Can you work these out from the model? Positions are in its coordinate system, mm. Face numbers are marked on the shaded views. A direction names the side the tool comes from. Coordinates: 2 decimals unless noted, no trailing zeros. Order: outer loops, then holes, each group sorted by start corner. A loop starts at its lowest first (then second) coordinate and runs counter-clockwise, first axis right, second up. Notation, with made-up numbers: (24, -1) -> (29, -1) arc R36 ccw to (29, 37) -> close; hole circle Ø4 at (39.5, 82). An arc over 180 degrees is marked (long way). Answer as a JSON object with one key per item and string values. Group by question number.
(1) I want a section at B-B, the plane z = 16.5. State how many separate pieces and enclosed holes the cut face has, plus the area to 3 significant figures.
(2) I want a section at D-D, the plane x = -65. List the corners of the cut face in (y, z) for me, plus the area to 3 significant figures.
(3) I want a section at A-A, the plane y = 0. List the corners of the cut face in (x, z) for me.
(4) For pin 1 (6 mm diameter, centred on y = -24, z = 4, fed in from -X); pin 2 (1 mm diameter, centred on y = 43, z = 8, fed in from -X); pin 3 (7 mm diameter, centred on x = 4, z = 4.5, fed in from +Y); pin 4 (5.5 mm diameter, centred on x = -55, y = -40, fed in from -Z), each with a flat end and sliding along its axis, tell me the tip position at first contact or that it passes through.
(5) I want a section at C-C, the plane x = 96.5. List the corners of the cut face in (y, z) for me, plus the area to 3 significant figures.
(6) I need wall thicknesses on line 1 (Y direction, x = 0.08, z = 15.75); line 2 (Y direction, x = -55, z = 10); line 3 (X direction, y = -9.5, z = 15.25). Which ranges of each line are inside material? Lowest first, please.
(7) If we mould it in two halves opening along Y, with no side actions, what happens to the marked faces 4, 5 and 6? For each: pulls with the +Y half, pulls with the -Y half, needs draft (parallel to the pull), parting line crosses it, or undercut.
(8) Which directions (+Z, -Z, +X, -X, +Y, -Y) give clear straight access to the entire face, cutting with the end or side of a thin tool? Please do the marked faces 1, 2 and 3.
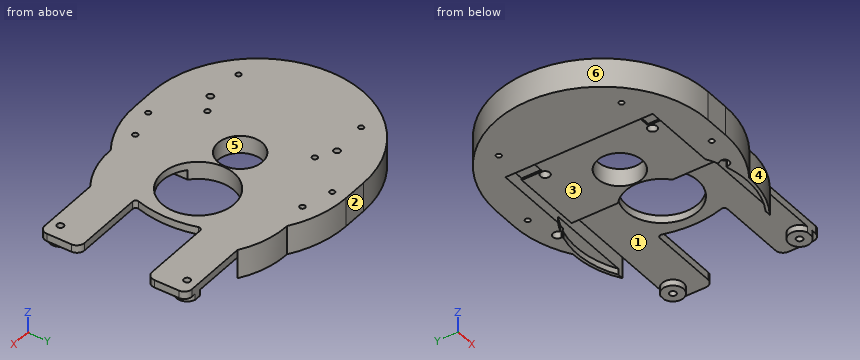
Autodesk Inventor part; units mm, degrees
ref_plane "YZ Plane" through (0, 0, 0) normal (1, 0, 0) x (0, 1, 0)
ref_plane "XZ Plane" through (0, 0, 0) normal (0, 1, 0) x (-1, 0, 0)
ref_plane "XY Plane" through (0, 0, 0) normal (0, 0, 1) x (1, 0, 0)
sketch "Sketch1" plane through (0, 0, 0) normal (0, 0, 1) x (1, 0, 0)
  line L0 (-19.2849, 35) -> (-19.2849, -35) construction
  line L1 (19.7114, 54.5) -> (19.7114, -54.5) construction
  line L2 (-19.2849, 35) -> (19.7114, 54.5) construction
  line L3 (-19.2849, -35) -> (19.7114, -54.5) construction
  circle A0 centre (0.08, 0) radius 14.5
  line L4 (-19.2849, 35) -> (0.08, 0) construction
  line L5 (0.08, 0) -> (-19.2849, -35) construction
  circle A1 centre (19.7114, 54.5) radius 1.75
  circle A2 centre (-19.2849, 35) radius 1.75
  circle A3 centre (-19.2849, -35) radius 1.75
  circle A4 centre (19.7114, -54.5) radius 1.75
  line L6 (-16, -69) -> (0, -69)
  line L7 (0, 69) -> (-16, 69)
  arc A5 (-16, 69) -> (-16, -69) centre (-16, 0) ccw
  arc A6 (0, -69) -> (0, 69) centre (0, 0) ccw
  line L8 (-85, 0) -> (69, 0) construction
  circle A7 centre (-19.2849, 35) radius 3
  circle A8 centre (-19.2849, -35) radius 3
  circle A9 centre (19.7114, 54.5) radius 3
  circle A10 centre (19.7114, -54.5) radius 3
  line L9 (0, -60) -> (0, 60) construction
  line L10 (-55, 40) -> (-55, -40) construction
  circle A11 centre (-55, 40) radius 1.65
  circle A12 centre (-55, -40) radius 1.65
  circle A13 centre (0, -60) radius 1.65
  circle A14 centre (0, 60) radius 1.65
  point P0 (-19.2849, 0)
  point P1 (19.7114, 0)
  point P2 (-55, 0)
  dimension "d0" = 70
  dimension "d1" = 109
  dimension "d2" = 43.6
  dimension "d3" = 29
  dimension "d4" = 40
  dimension "d5" = 3.5
  dimension "d7" = 138
  dimension "d8" = 154
  dimension "d33" = 6
  dimension "d55" = 85.08
  dimension "d110" = 120
  dimension "d111" = 30
  dimension "d112" = 80
  dimension "d113" = 3.3
extrude "Extrusion1" add sketch "Sketch1" along normal blind 19 contours A5 L7 A6 L6 | A7 | A8 | A9 | A10 | A11 | A12 | A13 | A14
sketch "Sketch2" plane through (0, 0, 19) normal (0, 0, 1) x (1, 0, 0)
  circle A0 centre (-52.47, 0) radius 18.5329 construction
  circle A1 centre (-71.0029, 0) radius 2
  circle A2 centre (-43.2035, 16.05) radius 2
  circle A3 centre (-43.2035, -16.05) radius 2
  circle A4 centre (0.08, 0) radius 14.5
  circle A5 centre (19.7114, -54.5) radius 1.75
  circle A6 centre (-19.2849, -35) radius 1.75
  circle A7 centre (-19.2849, 35) radius 1.75
  circle A8 centre (19.7114, 54.5) radius 1.75
  line L0 (-16, -69) -> (0, -69)
  arc A9 (0, -69) -> (0, 69) centre (0, 0) ccw
  line L1 (0, 69) -> (-16, 69)
  arc A10 (-16, 69) -> (-16, -69) centre (-16, 0) ccw
  arc A11 (-16, 69) -> (-16, -69) centre (-16, 0) ccw construction
  line L2 (-85, 0) -> (69, 0) construction
  circle A12 centre (-43.2035, -16.05) radius 5
  circle A13 centre (-43.2035, 16.05) radius 5
  circle A14 centre (-71.0029, 0) radius 5
  dimension "d11" = 120
  dimension "d12" = 120
  dimension "d13" = 32.1
  dimension "d14" = 52.55
  dimension "d40" = 4
  dimension "d49" = 10
sketch "Sketch3" plane through (0, 0, 0) normal (0, 0, -1) x (-1, 0, 0)
  circle A0 centre (30.8533, 41.3) radius 2.1
  circle A1 centre (-0.08, 0) radius 14.5
  circle A2 centre (30.8533, -41.3) radius 2.1
  line L0 (30.8533, 41.3) -> (-0.08, 0) construction
  line L1 (-0.08, 0) -> (30.8533, -41.3) construction
  circle A3 centre (-0.08, 0) radius 14.5 construction
  circle A4 centre (-19.7114, -54.5) radius 1.75 construction
  circle A5 centre (19.2849, -35) radius 1.75 construction
  circle A6 centre (19.2849, 35) radius 1.75 construction
  circle A7 centre (-19.7114, 54.5) radius 1.75 construction
  line L2 (16, -69) -> (0, -69) construction
  arc A8 (16, -69) -> (16, 69) centre (16, 0) ccw construction
  line L3 (0, 69) -> (16, 69) construction
  arc A9 (0, 69) -> (0, -69) centre (0, 0) ccw construction
  arc A10 (16, -69) -> (16, 69) centre (16, 0) ccw construction
  line L4 (85, 0) -> (-69, 0) construction
  arc A11 (0, 69) -> (0, -69) centre (0, 0) ccw construction
  line L5 (30.8533, 41.3) -> (30.8533, -41.3)
  line L6 (37.5533, 48) -> (-142.6467, 48)
  line L7 (-142.6467, 48) -> (-142.6467, -48)
  line L8 (-142.6467, -48) -> (37.5533, -48)
  line L9 (37.5533, -48) -> (37.5533, 48)
  line L10 (30.8533, 41.3) -> (37.5533, 41.3) construction
  line L11 (30.8533, 41.3) -> (30.8533, 48) construction
  line L12 (30.8533, -41.3) -> (37.5533, -41.3) construction
  line L13 (30.8533, -41.3) -> (30.8533, -48) construction
  circle A12 centre (-107.4467, 41.3) radius 2.1
  circle A13 centre (-107.4467, -41.3) radius 2.1
  line L14 (30.8533, 41.3) -> (-107.4467, 41.3) construction
  line L15 (30.8533, -41.3) -> (-107.4467, -41.3) construction
  line L16 (-23.4467, 48) -> (-23.4467, -48)
  circle A14 centre (-38.88, 0) radius 23.5
  circle A15 centre (-38.88, 0) radius 55.5
  arc A16 (-38.1482, 57.4953) -> (-70.5383, 48) centre (-38.88, 0) ccw
  arc A17 (-70.5383, -48) -> (-38.1482, -57.4953) centre (-38.88, 0) ccw
  line L17 (-38.1482, 57.4953) -> (-38.1482, 48)
  line L18 (-70.5383, 48) -> (-38.1482, 48)
  line L19 (-38.1482, -57.4953) -> (-38.1482, -48)
  line L20 (-70.5383, -48) -> (-38.1482, -48)
  dimension "d15" = 51.6
  dimension "d18" = 82.6
  dimension "d20" = 180.2
  dimension "d22" = 96
  dimension "d29" = 138.3
  dimension "d59" = 4.2
  dimension "d61" = 61
  dimension "d68" = 47
  dimension "d69" = 38.8
  dimension "d70" = 69
  dimension "d118" = 111
  dimension "d141" = 2
extrude "Extrusion14" cut sketch "Sketch3" against normal blind 14 contours L16 A14 L8 A15 L6 | L16 A14 | A15 L8 L7 L6 picked at (-49.8352, 39.5964) picked at (-36.3678, -0.9407)
extrude "Extrusion15" cut sketch "Sketch3" against normal blind 7.5 contours L6 A15 L8 L16 A14 | L6 L9 L8 A15 | A14 L16 picked at (-10.5973, 24.5754) picked at (-22.3115, -4.6826)
extrude "Extrusion16" cut sketch "Sketch3" against normal through all contours A0 | A2
sketch "Sketch8" plane through (0, 0, 19) normal (0, 0, 1) x (1, 0, 0)
  line L0 (-37.5533, 48) -> (-37.5533, -48)
  circle A0 centre (107.4467, -41.3) radius 2.1
  circle A1 centre (107.4467, 41.3) radius 2.1
  line L1 (-37.5533, -48) -> (117.4467, -48)
  line L2 (117.4467, -48) -> (117.4467, -22)
  line L3 (117.4467, -22) -> (-37.5533, -22)
  line L4 (-37.5533, -22) -> (-37.5533, -48)
  line L5 (49.5681, 48) -> (-37.5533, 48)
  line L6 (-37.5533, 48) -> (117.4467, 48)
  line L7 (117.4467, 48) -> (117.4467, 22)
  line L8 (117.4467, 22) -> (-37.5533, 22)
  line L9 (-37.5533, 22) -> (-37.5533, 48)
  circle A2 centre (107.4467, -41.3) radius 2.1
  circle A3 centre (107.4467, 41.3) radius 2.1
  arc A4 (109.474, -48) -> (105.4194, -48) centre (107.4467, -41.3) ccw
  arc A5 (105.4194, 48) -> (109.474, 48) centre (107.4467, 41.3) ccw
  point P0 (122.0315, -50.7282)
  point P1 (122.0315, 31.8718)
  dimension "d79" = 26
  dimension "d80" = 155
  dimension "d81" = 14
extrude "Extrusion18" add sketch "Sketch8" against normal up to surface (5 mm away)
extrude "Extrusion19" add sketch "Sketch8" against normal blind 9 contours L6 A5 | A4 L1
extrude "Extrusion17" cut sketch "Sketch3" against normal through all contours A14 L16 | L16 A14
extrude "Extrusion20" cut sketch "Sketch3" against normal through all contours A0 | A2
extrude "Extrusion21" cut sketch "Sketch1" along normal through all contours A2 | A3
extrude "Extrusion22" cut sketch "Sketch1" along normal blind 14 contours A7 | A8 | A9 | A10
extrude "Extrusion23" cut sketch "Sketch1" along normal through all contours A11 | A12 | A13 | A14
fillet "Fillet1" radius 5 1 edges at (117.4467, 48, 16.5)
fillet "Fillet2" radius 5 3 edges at (117.4467, 22, 16.5) (117.4467, -22, 16.5) (117.4467, -48, 16.5)
thread "Thread1"
thread "Thread2"
thread "Thread3"
thread "Thread4"
thread "Thread6"
thread "Thread7"
thread "Thread8"
thread "Thread9"
fillet "Fillet3" radius 2 2 edges at (65.3988, 22, 16.5) (65.3988, -22, 16.5)
extrude "Extrusion27" add sketch "Sketch3" against normal up to surface (19 mm away) contours L6 A15 L17 | L6 A16 L17 A15 | A15 L19 A17 L8 | L8 L19 A15 picked at (-54.2009, 49.4023) picked at (-54.2009, -49.4023)
extrude "Extrusion26" cut sketch "Sketch3" against normal blind 4 contours L16 A14 L8 A15 L6 | L6 L17 A15 | L6 A15 L8 L16 A14 | L6 A15 L17 | L8 L19 A15 | A15 L19 L8
chamfer "Chamfer2" distance 1 angle 45 4 edges at (22.2868, 52.9615, 2) (18.6661, 51.688, 2) (18.6661, -51.688, 2) (22.2868, -52.9615, 2)
sketch "Sketch10" plane through (0, 0, 7.5) normal (0, 0, -1) x (-1, 0, 0)
  line L0 (37.5533, 48) -> (37.5533, -48)
  line L1 (37.5533, 48) -> (22.5533, 48)
  line L2 (22.5533, 48) -> (22.5533, 34.5)
  line L3 (22.5533, 34.5) -> (37.5533, 34.5)
  line L4 (37.5533, 34.5) -> (37.5533, 48)
  line L5 (37.5533, -48) -> (22.5533, -48)
  line L6 (22.5533, -48) -> (22.5533, -34.5)
  line L7 (22.5533, -34.5) -> (37.5533, -34.5)
  line L8 (37.5533, -34.5) -> (37.5533, -48)
  point P0 (0, 0)
  dimension "d149" = 13.5
  dimension "d150" = 15
extrude "Extrusion29" cut sketch "Sketch10" against normal blind 1.2
properties part number "AZ-FLDIC-FWup top adapter"
Computed values:
{
 "1": {"separate pieces": "1", "enclosed holes": "14", "area": "18,000 mm2"},
 "2": {"outline": "(-48.58, 0) -> (48.58, 0) -> (48.58, 19) -> (-48.58, 19) -> close", "area": "1,850 mm2"},
 "3": {"outline": "(-85, 0) -> (-37.55, 0) -> (-37.55, 7.5) -> (-14.42, 7.5) -> (-14.42, 19) -> (-85, 19) -> close; (14.58, 7.5) -> (15.38, 7.5) -> (15.38, 19) -> (14.58, 19) -> close; (62.38, 14) -> (69, 14) -> (69, 19) -> (62.38, 19) -> close"},
 "4": {"pin 1": "stops at x = -81.73", "pin 2": "stops at x = -70.36", "pin 3": "stops at y = 69", "pin 4": "stops at z = 0"},
 "5": {"outline": "(-48, 14) -> (-22, 14) -> (-22, 19) -> (-48, 19) -> close; (22, 14) -> (48, 14) -> (48, 19) -> (22, 19) -> close", "area": "260 mm2"},
 "6": {"line 1": "y = -69 to -61.65, -58.35 to -14.5, 14.5 to 58.35, 61.65 to 69", "line 2": "y = -56.92 to -41.65, -38.35 to 38.35, 41.65 to 56.92", "line 3": "x = -84.34 to -10.87, 11.03 to 17.39, 60.37 to 68.34"},
 "7": {"face 4": "pulls with the -Y half", "face 5": "undercut", "face 6": "parting line crosses it"},
 "8": {"face 1": "-Z", "face 2": "+Z, -Z, +X, -X, +Y", "face 3": "-Z, +X"}
}
